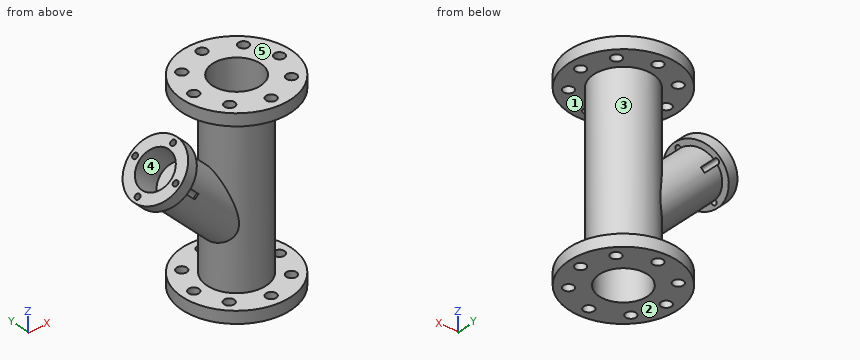
from build123d import *

# Parameters (mm, degrees)
F0_R      = 45
F1_DEPTH  = 10
F2_R      = 24.5
F3_DEPTH  = 140
F4_R      = 45.0356217661
F5_DEPTH  = 10
F6_R      = 20
F7_DEPTH  = 160
F8_R      = 4.25
F9_DEPTH  = 25
F10_R     = 4.25
F11_DEPTH = 25
F14_R     = 20
F15_DEPTH = 71.8
F16_R     = 25
F17_DEPTH = 10
F18_R     = 14.4589197706
F19_DEPTH = 98.5
F20_R     = 15.5945344816
F21_DEPTH = 25
F22_R     = 2.25
F23_DEPTH = 25


with BuildPart() as f1:
    # F0 (on Top) → F1 (new body)
    with BuildSketch(Plane.XY):
        Circle(F0_R)
    extrude(amount=F1_DEPTH)

    # F2 (on face) → F3 (join)
    with BuildSketch(Plane.XY.offset(10)):
        Circle(F2_R)
    extrude(amount=F3_DEPTH)

    # F4 (on face) → F5 (join)
    with BuildSketch(Plane.XY.offset(150)):
        Circle(F4_R)
    extrude(amount=F5_DEPTH)

    # F6 (on face) → F7 (cut)
    with BuildSketch(Plane(origin=(0, 0, 0), x_dir=(1, 0, 0), z_dir=(0, 0, -1))):
        Circle(F6_R)
    extrude(amount=-F7_DEPTH, mode=Mode.SUBTRACT)

    # F8 (on face) → F9 (cut)
    with BuildSketch(Plane.XY.offset(160)):
        with Locations((-25.2264022948, 24.2616699191)):
            Circle(F8_R)
        with Locations((25.2264022948, 24.2616699191)):
            Circle(F8_R)
        with Locations((0, 35)):
            Circle(F8_R)
        with Locations((35, 0)):
            Circle(F8_R)
        with Locations((25.7314957808, -23.7253055803)):
            Circle(F8_R)
        with Locations((0, -35)):
            Circle(F8_R)
        with Locations((-25.2264022948, -24.2616699191)):
            Circle(F8_R)
        with Locations((-35, 0)):
            Circle(F8_R)
    extrude(amount=-F9_DEPTH, mode=Mode.SUBTRACT)

    # F10 (on face) → F11 (cut)
    with BuildSketch(Plane(origin=(0, 0, 0), x_dir=(1, 0, 0), z_dir=(0, 0, -1))):
        with Locations((-25.4639357429, 24.0122463856)):
            Circle(F10_R)
        with Locations((0, 35)):
            Circle(F10_R)
        with Locations((25.4639357429, 24.0122463856)):
            Circle(F10_R)
        with Locations((35, 0)):
            Circle(F10_R)
        with Locations((25.4639357429, -24.0122463856)):
            Circle(F10_R)
        with Locations((0, -35)):
            Circle(F10_R)
        with Locations((-25.4639357429, -24.0122463856)):
            Circle(F10_R)
        with Locations((-35, 0)):
            Circle(F10_R)
    extrude(amount=-F11_DEPTH, mode=Mode.SUBTRACT)

    # F14 (on face) → F15 (join)
    with BuildSketch(Plane(origin=(-83.6396103068, 0, 83.6396103068), x_dir=(0.7071067812, 0, 0.7071067812), z_dir=(-0.7071067812, 0, 0.7071067812))):
        with Locations((34.390611576, 0)):
            Circle(F14_R)
    extrude(amount=-F15_DEPTH)

    # F16 (on face) → F17 (join)
    with BuildSketch(Plane(origin=(-83.6396103068, 0, 83.6396103068), x_dir=(0.7071067812, 0, 0.7071067812), z_dir=(-0.7071067812, 0, 0.7071067812))):
        with Locations((34.390611576, 0)):
            Circle(F16_R)
    extrude(amount=F17_DEPTH)

    # F18 (on face) → F19 (cut)
    with BuildSketch(Plane(origin=(-90.7106781187, 0, 90.7106781187), x_dir=(0.7071067812, 0, 0.7071067812), z_dir=(-0.7071067812, 0, 0.7071067812))):
        with Locations((34.390611576, 0)):
            Circle(F18_R)
    extrude(amount=F19_DEPTH, mode=Mode.SUBTRACT)

    # F20 (on face) → F21 (cut)
    with BuildSketch(Plane(origin=(-90.7106781187, 0, 90.7106781187), x_dir=(0.7071067812, 0, 0.7071067812), z_dir=(-0.7071067812, 0, 0.7071067812))):
        with Locations((34.390611576, 0)):
            Circle(F20_R)
    extrude(amount=-F21_DEPTH, mode=Mode.SUBTRACT)

    # F22 (on face) → F23 (cut)
    with BuildSketch(Plane(origin=(-90.7106781187, 0, 90.7106781187), x_dir=(0.7071067812, 0, 0.7071067812), z_dir=(-0.7071067812, 0, 0.7071067812))):
        with Locations((54.908573322, 0)):
            Circle(F22_R)
        with Locations((34.390611576, -20.517961746)):
            Circle(F22_R)
        with Locations((13.8726498301, 0)):
            Circle(F22_R)
        with Locations((34.390611576, 20.517961746)):
            Circle(F22_R)
    extrude(amount=-F23_DEPTH, mode=Mode.SUBTRACT)


solid = f1.part
Can you work these out from the model? Positions are in its coordinate system, mm. Face numbers are marked on the shaded views. A direction names the side the tool comes from. Give positions to 0.01 mm unless a question says otherwise; leave off trailing zeros. Loops run counter-clockwise (first coordinate to the right, second up) from the corner with the lowest first, then second, coordinate; pieces in that order, holes last. Notation, with made-up numbers: (69.25, -36.75) -> (122.25, -36.75) arc R15 ccw to (122.25, -30.75) -> close; hole circle Ø1 at (67.25, 52.5). An arc over 180 degrees is marked (long way). Use one line per item in the form item = value.
1) If we section it at A-A (z = 148): Please give me the cut outline in (x, y).
Answers:
outline = circle Ø49 at (0, 0); hole circle Ø40 at (0, 0)
2) If we section it at D-D (x = 0): Count the separate pieces of the cut face and the enclosed holes in it, plus the area to 3 significant figures.
Answers:
separate_pieces = 7
enclosed_holes = 0
area = 2,170 mm²
3) Will these pins go through, and if not, where does the flat tip stop? pin 1 (3 mm diameter, centred on x = -49, z = 92.5, fed in from -Y); pin 2 (1 mm diameter, centred on y = 5, z = 93.5, fed in from +X); pin 3 (1 mm diameter, centred on x = -58.5, y = 3.5, fed in from +Z).
Answers:
pin_1 = -19.89
pin_2 = 24.08
pin_3 = 88.07
4) For the marked faces 1 and 2, which set-ups out of +Z, -Z, +X, -X, +Y, -Y let a thin tool reach every point of the face, with its end or its side?
Answers:
face_1 = none
face_2 = -Z, +X, -X, +Y, -Y
5) We'd pull the mould along Y, two halves only. Please class the marked faces 3, 4 and 5: released by +Y, released by -Y, zero draft, split by the parting line, or undercut.
Answers:
face_3 = split by the parting line
face_4 = undercut
face_5 = zero draft
6) If we section it at B-B (y = -35): Please give me the cut outline in (x, z).
Answers:
outline = (-28.34, 150) -> (-4.25, 150) -> (-4.25, 160) -> (-28.34, 160) -> close; (-28.28, 0) -> (-4.25, 0) -> (-4.25, 10) -> (-28.28, 10) -> close; (4.25, 0) -> (28.28, 0) -> (28.28, 10) -> (4.25, 10) -> close; (4.25, 150) -> (28.34, 150) -> (28.34, 160) -> (4.25, 160) -> close
7) I need wall thicknesses on line 1 along Y through (x, z) = (0, 3); line 2 along Y through (x, z) = (1, 99.5); line 3 along Z through (x, y) = (39.5, 8.5). Which ranges of each line are inside material? Lowest first, please.
Answers:
line_1 = -45 to -39.25, -30.75 to -20, 20 to 30.75, 39.25 to 45
line_2 = -24.48 to -19.97, 19.97 to 24.48
line_3 = 0 to 10, 150 to 160
